For this review, take the finished solid that the model builds, in its own axes (mm). A direction names the side the tool comes from. Give positions to 0.01 mm unless a question says otherwise; leave off trailing zeros. Write each loop counter-clockwise with the first axis right and the second up, starting at its lowest first coordinate (ties: lowest second). Pieces come first, ordered by that corner, then holes.
from build123d import *

# Parameters (mm, degrees)
F1_DEPTH       = 12
F4_D           = 3.8
F4_DEPTH       = 40
F4_CSINK_D     = 8
F4_CSINK_ANGLE = 90
F5_SIZE        = 0.5


with BuildPart() as f1:
    # F0 (on Front) → F1 (new body)
    with BuildSketch(Plane.XZ):
        Polygon((-11, 0), (0, 0), (0, 3.6), (5.6, 3.6), (5.6, 2.1), (7.6, 2.1), (7.6, 5.1), (-11, 5.1), align=None)
    extrude(amount=F1_DEPTH)

    # F4
    with Locations(Plane.XY.offset(5.1)):
        with Locations((-5.5, -6)):
            CounterSinkHole(F4_D / 2, F4_CSINK_D / 2, depth=F4_DEPTH, counter_sink_angle=F4_CSINK_ANGLE)

    # F5
    f5_edges = [f1.edges().sort_by_distance(p)[0] for p in [
        (-1.7, -12, 5.1),
        (7.6, -6, 5.1),
        (-1.7, 0, 5.1),
        (-11, -6, 5.1),
        (-11, -12, 2.55),
        (-11, 0, 2.55),
        (7.6, 0, 3.6),
        (7.6, -12, 3.6),
        (0, -12, 1.8),
        (5.6, -12, 2.85),
        (0, 0, 1.8),
        (5.6, 0, 2.85),
    ]]
    chamfer(f5_edges, length=F5_SIZE)


solid = f1.part
(1) We need section A-A (x = -5.5). Write out the cut boundary in (y, z).
(2) The part is to be moulded in two halves that separate along X. For faces 1 (the flat face through (-11, -6, 2)), 2 (the flat face through (-4, -12, 3)), 3 (the flat face through (5.6, -6, 3)), say which applies: +X half, -X half, draft (parallel to the pull), parting line (faces both ways), or undercut.
(3) We need section C-C (y = -6). Write out the cut boundary in (x, z), and give its area (3 significant figures).
(4) We need section B-B (z = 4.15). Write out the cut boundary in (x, y), and give its area (3 significant figures).
(5) Tool access review of faces 4 (the flat face through (0, -6, 2)), 5 (the flat face through (0, -6, 5.1)), 6 (the flat face through (7, -6, 2.1)): name each direction out of +Z, -Z, +X, -X, +Y, -Y from which nothing blocks a thin tool from reaching the whole face with its end or side.
(6) Clearance check with flat-ended pins moving along their axes: pin 1 Ø0.6 at (x, y) = (7, -8) entering from -Z; pin 2 Ø2 at (x, y) = (2, -9) entering from -Z; pin 3 Ø4.5 at (x, y) = (-5.5, -6) entering from +Z. State where each tip first meets the part, or that it passes through.
(7) For L1, parallel to X at y = -6, z = 2.4; L2, parallel to X at y = -6, z = 1.95; L3, parallel to Y at x = -5.5, z = 1.7, list the stretches that pass through material, from the lowest coordinate up.
(8) We need section D-D (x = 0.25). Write out the cut boundary in (y, z), and give its area (4 significant figures).
The answers:
1. outline: (-12, 0) - (-7.9, 0) - (-7.9, 3) - (-10, 5.1) - (-11.5, 5.1) - (-12, 4.6) - close; (-4.1, 0) - (0, 0) - (0, 4.6) - (-0.5, 5.1) - (-2, 5.1) - (-4.1, 3) - close
2. face 1: -X half
2. face 2: draft
2. face 3: undercut
3. outline: (-11, 0) - (-7.4, 0) - (-7.4, 3) - (-9.5, 5.1) - (-10.5, 5.1) - (-11, 4.6) - close; (-3.6, 0) - (0, 0) - (0, 3.6) - (5.6, 3.6) - (5.6, 2.1) - (7.6, 2.1) - (7.6, 4.6) - (7.1, 5.1) - (-1.5, 5.1) - (-3.6, 3) - close
3. area: 46.5 mm2
4. outline: (-11, -11.5) - (-10.5, -12) - (7.1, -12) - (7.6, -11.5) - (7.6, -0.5) - (7.1, 0) - (-10.5, 0) - (-11, -0.5) - close; hole circle Ø6.1 at (-5.5, -6)
4. area: 193 mm2
5. face 4: -Z, +Y, -Y
5. face 5: +Z, +X, -X, +Y, -Y
5. face 6: -Z, +X, +Y, -Y
6. pin 1: stops at z = 2.1
6. pin 2: stops at z = 3.6
6. pin 3: stops at z = 3.35
7. L1: x = -11 to -7.4, -3.6 to 0, 5.6 to 7.6
7. L2: x = -11 to -7.4, -3.6 to 0
7. L3: y = -12 to -7.9, -4.1 to 0
8. outline: (-12, 3.6) - (0, 3.6) - (0, 4.6) - (-0.5, 5.1) - (-11.5, 5.1) - (-12, 4.6) - close
8. area: 17.75 mm2
